Check sheet for the modelled part. Datum: model origin and axes. Units: mm. Give positions to 0.01 mm unless a question says otherwise; leave off trailing zeros. Order: outer loops, then holes, each group sorted by start corner. A loop starts at its lowest first (then second) coordinate and runs counter-clockwise, first axis right, second up. Notation, with made-up numbers: M 72.25,-38.5 L 97.25,-38.5 A35 cw 97.25,-2.5 Z; hole C -13,16 d9. An arc over 180 degrees is marked long. Answer in a Markdown table with one row per item. Add a question column.
from build123d import *

# Parameters (mm, degrees)
F0_W     = 44.45
F0_H     = 44.45
F1_DEPTH = 44.45
F2_SIZE  = 1.905
F4_DEPTH = 25.4
F5_W     = 38.1
F5_H     = 38.1
F6_DEPTH = 38.1
F7_SIZE  = 2.54


with BuildPart() as f1:
    # F0 (on Top) → F1 (new body)
    with BuildSketch(Plane.XY):
        with Locations((1.98498182, -0.7634516805)):
            Rectangle(F0_W, F0_H)
    extrude(amount=F1_DEPTH)

    # F2
    f2_edges = [f1.edges().sort_by_distance(p)[0] for p in [
        (-20.240018, -22.988452, 22.225),
        (1.984982, -22.988452, 0),
        (-20.240018, -0.763452, 0),
    ]]
    chamfer(f2_edges, length=F2_SIZE)

    # F3 (on face) → F4 (join)
    with BuildSketch(Plane(origin=(-13.1394899535, -13.1394899535, -13.1394899535), x_dir=(0.8164965809, -0.4082482905, -0.4082482905), z_dir=(-0.5773502692, -0.5773502692, -0.5773502692))):
        with BuildLine():
            Line((-8.6963355296, 16.2552900723), (-7.5297660396, 16.9288092814))
            Line((-7.5297660396, 16.9288092814), (-6.3631965496, 17.6023284905))
            Line((-6.3631965496, 17.6023284905), (-12.2885202748, 27.8652902339))
            ThreePointArc((-12.2885202748, 27.8652902339), (-13.4909095429, 27.2538127004), (-14.6216592548, 26.5182518157))
            Line((-14.6216592548, 26.5182518157), (-8.6963355296, 16.2552900723))
        make_face()
        with BuildLine():
            Line((-6.3631965496, 17.6023284905), (-7.1409095429, 16.2552900723))
            Line((-7.1409095429, 16.2552900723), (-8.6963355296, 16.2552900723))
            Line((-8.6963355296, 16.2552900723), (-14.6216592548, 26.5182518157))
            ThreePointArc((-14.6216592548, 26.5182518157), (-12.8978392219, 4.935053296), (5.5590904571, 16.2552900723))
            ThreePointArc((5.5590904571, 16.2552900723), (-0.2157617573, 26.9010558103), (-12.2885202748, 27.8652902339))
            Line((-12.2885202748, 27.8652902339), (-6.3631965496, 17.6023284905))
        make_face()
        Polygon((-7.1409095429, 16.2552900723), (-7.5297660396, 16.9288092814), (-8.6963355296, 16.2552900723), align=None)
        Polygon((-6.3631965496, 17.6023284905), (-7.5297660396, 16.9288092814), (-7.1409095429, 16.2552900723), align=None)
    extrude(amount=-F4_DEPTH)

    # F5 (on face) → F6 (cut)
    with BuildSketch(Plane.YZ.offset(24.20998182)):
        with Locations((2.4115483195, 25.4)):
            Rectangle(F5_W, F5_H)
    extrude(amount=-F6_DEPTH, mode=Mode.SUBTRACT)

    # F7 (call 1 of 4: OpenCascade refuses the feature's edges together)
    f7_edges = [f1.edges().sort_by_distance(p)[0] for p in [
        (-20.240018, 21.461548, 23.1775),
        (-20.240018, 0.189048, 44.45),
    ]]
    chamfer(f7_edges, length=F7_SIZE)

    # F7#2 (call 2 of 4)
    f7_2_edges = [f1.edges().sort_by_distance(p)[0] for p in [
        (2.937482, 21.461548, 0),
        (24.209982, 0.189048, 0),
    ]]
    chamfer(f7_2_edges, length=F7_SIZE)

    # F7#3 (call 3 of 4)
    f7_3_edges = [f1.edges().sort_by_distance(p)[0] for p in [
        (2.937482, -22.988452, 44.45),
        (24.209982, -22.988452, 23.1775),
    ]]
    chamfer(f7_3_edges, length=F7_SIZE)

    # F7#4 (call 4 of 4)
    f7_4_edges = [f1.edges().sort_by_distance(p)[0] for p in [
        (5.159982, 21.461548, 6.35),
        (24.209982, 2.411548, 6.35),
        (24.209982, -16.638452, 25.4),
        (5.159982, -16.638452, 44.45),
        (-13.890018, 2.411548, 44.45),
        (-13.890018, 21.461548, 25.4),
    ]]
    chamfer(f7_4_edges, length=F7_SIZE)


solid = f1.part
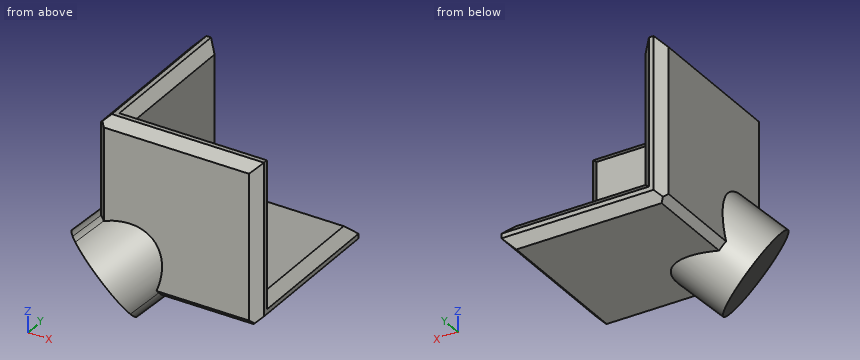
Q1. Cross-section at B-B (y = 15). Record the boundary of the cut face in (x, z) (3 decimals).
Q2. Go/stop test with flat-tipped pins: pin 1 (8 mm diameter, centred on x = 17.5, y = -4.5, fed in from -Z); pin 2 (8 mm diameter, centred on x = -17, z = 1, fed in from -Y); pin 3 (4 mm diameter, centred on y = -8.5, z = 27, fed in from -X). Record where each tip stops, or that it passes through.
Q3. Cross-section at A-A (z = 19). Record the boundary of the cut face in (x, y).
Q4. Thickness scan on probe 1 along Y at (x, z) = (17, 29); probe 2 along X at (y, z) = (-10.5, 35); probe 3 along Z at (x, y) = (11, -6). Record the ranges inside material, lowest first.
Values follow:
| question | item | result |
|---|---|---|
| 1 | outline | M -20.24,1.905 L -18.335,0 L 21.67,0 L 24.21,2.54 L 24.21,3.81 L 21.67,6.35 L -13.89,6.35 L -13.89,41.91 L -16.43,44.45 L -17.7,44.45 L -20.24,41.91 Z |
| 2 | pin 1 | z = 0 |
| 2 | pin 2 | y = -29.08 |
| 2 | pin 3 | x = -20.24 |
| 3 | outline | M -20.24,-21.08 L -18.34,-22.99 L 21.67,-22.99 L 24.21,-20.45 L 24.21,-19.18 L 21.67,-16.64 L -13.89,-16.64 L -13.89,18.92 L -16.43,21.46 L -17.7,21.46 L -20.24,18.92 Z |
| 4 | probe 1 | -22.99 to -16.64 |
| 4 | probe 2 | -20.24 to -13.89 |
| 4 | probe 3 | 0 to 6.35 |
